Source: CAD feature listing. Evaluate the final solid. Frame: model axes, mm. Face numbers are marked on the shaded views. Round coordinates to 2 decimals unless told otherwise and drop trailing zeros. Loops run counter-clockwise (first coordinate to the right, second up) from the corner with the lowest first, then second, coordinate; pieces in that order, holes last. Notation, with made-up numbers: M 45,50.5 L 80,50.5 A22 ccw 80,86.5 Z; hole C 57.25,66 d1. An arc over 180 degrees is marked long. One line per item, written item: value.
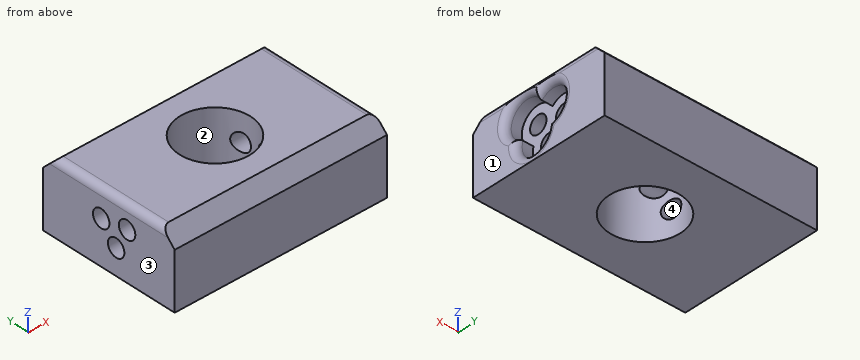
from build123d import *

# Parameters (mm, degrees)
F0_W           = 76.2
F0_H           = 50.8
F0_R           = 12.7
F1_DEPTH       = 25.4
F3_D           = 6.35
F3_CBORE_D     = 12.7
F3_CBORE_DEPTH = 6.35
F4_SIZE        = 5.08
F5_R           = 2.54
F6_T1_DEPTH    = 53.34
F6_T4_ANGLE    = 333.5496050311
F6_T6_ANGLE    = 313.8522207809
F6_T8_ANGLE    = 339.5771348814


# Not quite as in the source:
# - a fillet or chamfer that OpenCascade refuses, or shapes differently, is made with other operations: its cross-section is extruded or revolved along the edge and cut away or added


with BuildPart() as f1:
    # F0 (on Top) → F1 (new body)
    with BuildSketch(Plane.XY):
        Rectangle(F0_W, F0_H)
        Circle(F0_R, mode=Mode.SUBTRACT)
    extrude(amount=F1_DEPTH)

    # F3 (through all)
    with Locations(Plane.YZ.offset(38.1)):
        with Locations((-7.0466324687, 17.1319264919), (2.941543702, 15.6153971329), (-2.8108085971, 9.1309268028)):
            CounterBoreHole(F3_D / 2, F3_CBORE_D / 2, F3_CBORE_DEPTH)

    # F4
    f4_edges = [f1.edges().sort_by_distance(p)[0] for p in [
        (0, -25.4, 25.4),
        (0, 25.4, 25.4),
    ]]
    chamfer(f4_edges, length=F4_SIZE)

    # F5
    f5_edges = [f1.edges().sort_by_distance(p)[0] for p in [
        (-38.1, 0, 25.4),
    ]]
    fillet(f5_edges, radius=F5_R)

    # F6: fillet of radius 2.54 on 4 edges, made by hand

    # F6_s2 → F6_t1 (cut)
    with BuildSketch(Plane.XZ.offset(-26.67)):
        with BuildLine():
            ThreePointArc((35.56, 25.4), (37.3560512242, 24.6560512242), (38.1, 22.86))
            Line((38.1, 22.86), (38.1, 25.4))
            Line((38.1, 25.4), (35.56, 25.4))
        make_face()
    extrude(amount=F6_T1_DEPTH, mode=Mode.SUBTRACT)

    # F6_s3 → F6_t4 (revolve, cut)
    with BuildSketch(Plane(origin=(0, -6.4599960512, 8.2833530872), x_dir=(1, 0, 0), z_dir=(0, -0.6149714639, 0.7885493634))):
        with BuildLine():
            ThreePointArc((38.1, 3.032576048), (37.3560512242, 4.8286272723), (35.56, 5.572576048))
            Line((35.56, 5.572576048), (38.1, 5.572576048))
            Line((38.1, 5.572576048), (38.1, 3.032576048))
        make_face()
    revolve(axis=Axis((38.1, 2.941543702, 15.6153971329), (1, 0, 0)), revolution_arc=F6_T4_ANGLE, mode=Mode.SUBTRACT)

    # F6_s5 → F6_t6 (revolve, cut)
    with BuildSketch(Plane(origin=(0, -0.3361656341, -0.0902154954), x_dir=(1, 0, 0), z_dir=(0, 0.9658250629, 0.2591948067))):
        with BuildLine():
            ThreePointArc((38.1, -18.4374249449), (37.3560512242, -16.6413737207), (35.56, -15.8974249449))
            Line((35.56, -15.8974249449), (38.1, -15.8974249449))
            Line((38.1, -15.8974249449), (38.1, -18.4374249449))
        make_face()
    revolve(axis=Axis((38.1, -2.8108085971, 9.1309268028), (1, 0, 0)), revolution_arc=F6_T6_ANGLE, mode=Mode.SUBTRACT)

    # F6_s7 → F6_t8 (revolve, cut)
    with BuildSketch(Plane(origin=(0, 5.5955772378, 10.1893133195), x_dir=(1, 0, 0), z_dir=(0, -0.4813542865, -0.8765261267))):
        with BuildLine():
            ThreePointArc((38.1, 5.5330837175), (37.3560512242, 7.3291349418), (35.56, 8.0730837175))
            Line((35.56, 8.0730837175), (38.1, 8.0730837175))
            Line((38.1, 8.0730837175), (38.1, 5.5330837175))
        make_face()
    revolve(axis=Axis((38.1, -7.0466324687, 17.1319264919), (1, 0, 0)), revolution_arc=F6_T8_ANGLE, mode=Mode.SUBTRACT)


solid = f1.part
1. Section query B-B (x = -17.5). Return the cut outline in (y, z) (3 decimals).
Report:
outline: M -25.4,0 L 25.4,0 L 25.4,20.32 L 20.32,25.4 L -20.32,25.4 L -25.4,20.32 Z; hole C -7.047,17.132 d6.35; hole C -2.811,9.131 d6.35; hole C 2.942,15.615 d6.35
2. Pull-direction query (X, two-part tool) for the marked faces 1, 2, 3 and 4; classes: released by +X, released by -X, zero draft, split by the parting line, or undercut.
Report:
face 1: released by +X
face 2: undercut
face 3: released by -X
face 4: zero draft
3. Section query A-A (x = 0). Return the cut outline in (y, z), and give its area (3 significant figures).
Report:
outline: M -25.4,0 L -12.7,0 L -12.7,25.4 L -20.32,25.4 L -25.4,20.32 Z; M 12.7,0 L 25.4,0 L 25.4,20.32 L 20.32,25.4 L 12.7,25.4 Z
area: 619 mm2
4. Pin query (flat end, axial travel): pin 1 (5 mm diameter, centred on y = -2.81, z = 9.13, fed in from -X) (3 decimals); pin 2 (8 mm diameter, centred on y = -3.5, z = 18, fed in from +X). Return the tip coordinate at first contact, or that it passes through.
Report:
pin 1: passes through
pin 2: stops at x = 37.39
5. Ray query, line 1 (Y direction, x = -22, z = 11.5); line 2 (Y direction, x = -27.5, z = 9.5); line 3 (X direction, y = 8, z = 11). Return the intervals inside material, ascending. Write a range as [from, to].
Report:
line 1: y = [-25.4, -4.92], [-0.7, 25.4]
line 2: y = [-25.4, -5.96], [0.34, 25.4]
line 3: x = [-38.1, -9.86], [9.86, 37.07]
